from build123d import *

# Parameters (mm, degrees)
BOSS_EXTRUDE1_DEPTH      = 3.175
BOSS_EXTRUDE1_DEPTH_BACK = 3.175
SKETCH1_W                = 110
SKETCH1_H                = 85
SKETCH1_R                = 2.25
SKETCH1_R_2              = 2.5


with BuildPart() as part:
    # Sketch1 → Boss-Extrude1 (new, two sides: drawn at the far end of the back side and taken through both)
    with BuildSketch(Plane(origin=(0, 0, 0), x_dir=(1, 0, 0), z_dir=(0, 1, 0)).offset(-BOSS_EXTRUDE1_DEPTH_BACK)):
        Rectangle(SKETCH1_W, SKETCH1_H)
        with Locations(Location((-45.5, 22.5, 0), (0, 0, 270))):
            Circle(SKETCH1_R, mode=Mode.SUBTRACT)
        with Locations(Location((45.5, 22.5, 0), (0, 0, 90))):
            Circle(SKETCH1_R, mode=Mode.SUBTRACT)
        with Locations(Location((45.5, -22.5, 0), (0, 0, 270))):
            Circle(SKETCH1_R, mode=Mode.SUBTRACT)
        with Locations(Location((-45.5, -22.5, 0), (0, 0, 90))):
            Circle(SKETCH1_R, mode=Mode.SUBTRACT)
        with Locations(Location((45, -32.5, 0), (0, 0, 270))):
            Circle(SKETCH1_R_2, mode=Mode.SUBTRACT)
        with Locations(Location((-45, -32.5, 0), (0, 0, 90))):
            Circle(SKETCH1_R_2, mode=Mode.SUBTRACT)
        with Locations(Location((-45, 32.5, 0), (0, 0, 270))):
            Circle(SKETCH1_R_2, mode=Mode.SUBTRACT)
        with Locations(Location((45, 32.5, 0), (0, 0, 90))):
            Circle(SKETCH1_R_2, mode=Mode.SUBTRACT)
        with Locations(Location((0, -32.5, 0), (0, 0, 270))):
            Circle(SKETCH1_R_2, mode=Mode.SUBTRACT)
        with Locations(Location((0, 32.5, 0), (0, 0, 270))):
            Circle(SKETCH1_R_2, mode=Mode.SUBTRACT)
    extrude(amount=BOSS_EXTRUDE1_DEPTH + BOSS_EXTRUDE1_DEPTH_BACK)


solid = part.part
Model file for the job. Use its own axes, mm. Give positions to 0.01 mm unless a question says otherwise; leave off trailing zeros. Loops run counter-clockwise (first coordinate to the right, second up) from the corner with the lowest first, then second, coordinate; pieces in that order, holes last. Notation, with made-up numbers: (-37.75, 61) - (-25.75, 61) arc R6 ccw to (-25.75, 65) - close; hole circle Ø2 at (9, 39.5). An arc over 180 degrees is marked (long way). Use one line per item in the form item = value.
(1) Cut at A-A (z = -32.5). Give the cut face in (x, y) (3 decimals).
Determined:
outline = (-55, -3.175) - (-47.5, -3.175) - (-47.5, 3.175) - (-55, 3.175) - close; (-42.5, -3.175) - (-2.5, -3.175) - (-2.5, 3.175) - (-42.5, 3.175) - close; (2.5, -3.175) - (42.5, -3.175) - (42.5, 3.175) - (2.5, 3.175) - close; (47.5, -3.175) - (55, -3.175) - (55, 3.175) - (47.5, 3.175) - close
(2) Drill centre lines: L1, parallel to X at y = -1, z = 32.5; L2, parallel to X at y = -2.25, z = -24; L3, parallel to Z at x = 44, y = 2.5. Where is each one in solid material? Low to high.
Determined:
L1 = -55 to -47.5, -42.5 to -2.5, 2.5 to 42.5, 47.5 to 55
L2 = -55 to -47.18, -43.82 to 43.82, 47.18 to 55
L3 = -42.5 to -34.79, -30.21 to -24.18, -20.82 to 20.82, 24.18 to 30.21, 34.79 to 42.5
(3) Cut at B-B (y = -1.75). Count the separate pieces of the cut face and the enclosed holes in it, then the cut area to 3 significant figures.
Determined:
separate_pieces = 1
enclosed_holes = 10
area = 9,170 mm^2
(4) Pull direction Z, two halves, no side cores. Call faces 1 (the face through (-1, 3.175, -1)), 2 (the face through (-43.603, -0.044, -21.29)), 3 (the face through (-1, 0, 42.5)): pulls with the +Z half, pulls with the -Z half, needs draft (parallel to the pull), parting line crosses it, or undercut.
Determined:
face_1 = needs draft
face_2 = undercut
face_3 = pulls with the +Z half
